For this review, take the finished solid that the model builds, in its own axes (mm). A direction names the side the tool comes from. Coordinates: 2 decimals unless noted, no trailing zeros. Answer as a JSON object with one key per item and string values. Group by question number.
1) Machinability: for faces 4 (the cylindrical face through (86.99, -23.59, 29.62)), 5 (the flat face through (79, 17, 3.175)), which of the approach directions +Z, -Z, +X, -X, +Y, -Y give a long, thin tool a straight path to every point of the face, cutting with its end or side? Answer none if there is none.
2) For pin 1 (6.5 mm diameter, centred on x = -78, y = 14.5, fed in from -Z) (3 decimals), flat-tipped, find the tip position at first contact; note if it passes through.
3) Wall thickness on L1, parallel to X at y = -21, z = 52.5: over which ranges is the line inside the solid? List them lowest first.
4) Draft analysis for pull direction Y (two halves, no side actions). For faces 1 (the flat face through (-1, 25.4, 29)), 2 (the cylindrical face through (-73.318, 14.857, 1.565)), 3 (the flat face through (-88.9, 0, 29)), state which applies: +Y half, -Y half, draft (parallel to the pull), parting line (faces both ways), or undercut.
from build123d import *

# Parameters (mm, degrees)
F0_W     = 177.8
F0_H     = 50.8
F1_DEPTH = 58.42
F2_R     = 6.35
F3_R     = 6.35
F4_DEPTH = 3.175


with BuildPart() as f1:
    # F0 (on Top) → F1 (new body)
    with BuildSketch(Plane.XY):
        Rectangle(F0_W, F0_H)
    extrude(amount=F1_DEPTH)

    # F2
    f2_edges = [f1.edges().sort_by_distance(p)[0] for p in [
        (-88.9, 25.4, 29.21),
        (88.9, 25.4, 29.21),
        (88.9, -25.4, 29.21),
        (-88.9, -25.4, 29.21),
    ]]
    fillet(f2_edges, radius=F2_R)

    # F3 (on face) → F4 (cut)
    with BuildSketch(Plane(origin=(0, 0, 0), x_dir=(1, 0, 0), z_dir=(0, 0, -1))):
        with Locations((79.375, 16.764)):
            Circle(F3_R)
        with Locations((79.375, -16.764)):
            Circle(F3_R)
        with Locations((-79.375, 16.764)):
            Circle(F3_R)
        with Locations((-79.375, -16.764)):
            Circle(F3_R)
    extrude(amount=-F4_DEPTH, mode=Mode.SUBTRACT)


solid = f1.part
Output values:
{
 "1": {"face 4": "+Z, -Z, +X, -Y", "face 5": "-Z"},
 "2": {"pin 1": "stops at z = 3.175"},
 "3": {"L1": "x = -88.59 to 88.59"},
 "4": {"face 1": "+Y half", "face 2": "undercut", "face 3": "draft"}
}
